```python
from build123d import *

# Parameters (mm, degrees)
F1_DEPTH = 3


with BuildPart() as f1:
    # F0 (on Top) → F1 (new body)
    with BuildSketch(Plane.XY):
        Polygon((-112.955246, -3.54154), (-118.796036, 11.650806), (-124.313387, -3.151842), (-141.807427, -3.151842), (-127.879479, -12.571709), (-134.473386, -27.710782), (-130.965268, -25.908628), (-132.387559, -29.796608), (-152.707559, -29.796608), (-152.799174, -41.2316), (-137.323676, -41.2316), (-144.994139, -65.857825), (-138.929132, -66.758923), (-132.882882, -41.2316), (-130.178067, -41.231918), (-135.287017, -66.759351), (-129.549282, -67.969184), (-125.885266, -41.2316), (-123.340191, -41.2319), (-125.867149, -69.316173), (-120.080659, -73.319617), (-119.616715, -41.2316), (-116.949647, -41.231914), (-116.949647, -72.583164), (-110.730788, -68.840947), (-113.186582, -41.2316), (-110.90286, -41.2316), (-106.963308, -68.292474), (-101.254005, -66.865148), (-106.145109, -41.2316), (-104.622629, -41.2316), (-97.828425, -66.865148), (-91.776701, -65.36576), (-99.484258, -41.2316), (-84.710565, -41.2319), (-84.749944, -29.796608), (-102.529944, -29.796608), (-105.977231, -25.908628), (-102.963967, -27.996385), (-109.339354, -12.390961), (-95.637031, -3.54154), align=None)
        Polygon((-129.171015, -29.796608), (-127.458225, -23.673594), (-125.715271, -22.778221), (-127.315492, -29.796608), align=None, mode=Mode.SUBTRACT)
        Polygon((-123.927363, -29.709139), (-122.748051, -20.676211), (-121.729279, -20.152858), (-122.224698, -29.796608), align=None, mode=Mode.SUBTRACT)
        Polygon((-119.167684, -29.796403), (-118.796036, -18.202179), (-117.97959, -18.506491), (-117.419369, -29.796608), align=None, mode=Mode.SUBTRACT)
        Polygon((-114.562619, -29.796413), (-115.040493, -20.152858), (-112.898951, -21.204401), (-112.899961, -29.796608), align=None, mode=Mode.SUBTRACT)
        Polygon((-110.19575, -29.796608), (-110.194964, -23.110219), (-108.188545, -24.591885), (-108.028096, -29.796608), align=None, mode=Mode.SUBTRACT)
    extrude(amount=F1_DEPTH)


solid = f1.part
```
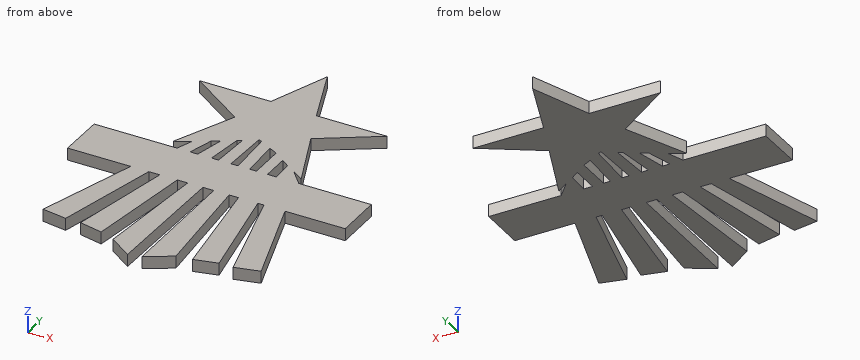
Geometry check sheet. Reference: the model listing, model coordinates, mm. Coordinates: 2 decimals unless noted, no trailing zeros. Write each loop counter-clockwise with the first axis right and the second up, starting at its lowest first coordinate (ties: lowest second). Pieces come first, ordered by that corner, then holes. Notation, with made-up numbers: (61.5, 73) -> (80.5, 73) arc R8 ccw to (80.5, 83) -> close; hole circle Ø3 at (-30, 17). An arc over 180 degrees is marked (long way). Use CSV: the item, a comma, the result in double quotes. Start each with the question number.
Item 1: Thickness scan on line 1 (X direction, y = -45, z = 0.5); line 2 (X direction, y = -51, z = 0.9); line 3 (X direction, y = -19.5, z = 0.55). Record the ranges inside material, lowest first.
Item 2: Depth check by flat-ended pin: pin 1 Ø1.4 at (x, z) = (-131, 2) entering from -Y; pin 2 Ø0.9 at (y, z) = (-28, 2) entering from +X; pin 3 Ø1.5 at (x, z) = (-108, 0.5) entering from +Y. Enter the tip coordinate at first touch or a pass-through.
Item 3: Cross-section at A-A, the plane x = -144. Record the cut outline in (y, z), plus the area to 3 significant figures.
Item 4: Cross-section at B-B, the plane z = 0.7. State how many separate pieces and enclosed holes the cut face has, plus the area to 3 significant figures.
Item 5: Cross-section at C-C, the plane y = -0.5. Record the cut outline in (x, z).
Answers:
1,line 1,"-138.5 to -133.78, -130.93 to -126.4, -123.68 to -119.67, -116.95 to -112.85, -110.35 to -105.43, -103.62 to -98.28"
1,line 2,"-140.37 to -135.2, -132.13 to -127.22, -124.22 to -119.76, -116.95 to -112.32, -109.48 to -104.28, -102.03 to -96.36"
1,line 3,"-130.9 to -118.84, -117.93 to -106.44"
2,pin 1,"y = -67.81"
2,pin 2,"x = -102.96"
2,pin 3,"y = -3.54"
3,outline,"(-66.01, 0) -> (-62.67, 0) -> (-62.67, 3) -> (-66.01, 3) -> close; (-41.23, 0) -> (-29.8, 0) -> (-29.8, 3) -> (-41.23, 3) -> close"
3,area,"44.3 mm^2"
4,separate pieces,"1"
4,enclosed holes,"5"
4,area,"2,380 mm^2"
5,outline,"(-123.32, 0) -> (-114.12, 0) -> (-114.12, 3) -> (-123.32, 3) -> close"
